Read the model definition and answer for the solid it produces. Units are mm, in the model's axes. A direction names the side the tool comes from. Give positions to 0.01 mm unless a question says otherwise; leave off trailing zeros. Order: outer loops, then holes, each group sorted by start corner. A loop starts at its lowest first (then second) coordinate and runs counter-clockwise, first axis right, second up. Notation, with made-up numbers: (-38.5, 2) -> (-1.5, 2) arc R24 ccw to (-1.5, 14) -> close; hole circle Ø6 at (-4, -15). An arc over 180 degrees is marked (long way). Answer as CSV lines item,"result". Start each with the question number.
1) Straight lines are drawn through the part: L1, parallel to X at y = 0, z = 48.5; L2, parallel to Y at x = 237.5, z = 21.5; L3, parallel to X at y = -32, z = 38. For each, find the intervals that lie inside material, in ascending order. Write a range as from..to.
2) Find section A-A (x = 0). Determine the outline of the cut face in (y, z), and give its area (3 significant figures).
3) The mould has two halves that part along Z. Classify faces 1 (the face through (278.814, 31.839, 41.915)), 2 (the face through (246, -25.4, 38)), 3 (the face through (284.86, -31.66, 20.34)): +Z half, -Z half, draft (parallel to the pull), parting line (faces both ways), or undercut.
4) Find section C-C (x = 228). Determine the outline of the cut face in (y, z), and give its area (3 significant figures).
5) Find section B-B (z = 6.5). Determine the outline of the cut face in (x, y).
6) For faces 4 (the face through (43.272, -16.365, 37.744)), 5 (the face through (237, 38.1, 38)), 6 (the face through (122, -23, 31.75)), 7 (the face through (215.9, 0, 38)), determine the directions among +Z, -Z, +X, -X, +Y, -Y from which every point of the face is accessible in a straight line to the end or side of a thin tool.
7) Find section D-D (y = -44.5). Determine the outline of the cut face in (x, z).
8) Flat-ended cylindrical pins translate along their axes: pin 1 Ø5 at (y, z) = (-10.5, 18.5) entering from -X; pin 2 Ø7.5 at (y, z) = (24.5, 28.5) entering from -X; pin 3 Ø15 at (y, z) = (3.5, 34.5) entering from +X. Find the tip coordinate at first contact, or state that the pin passes through.
```python
from build123d import *
from build123d import SkipClean  # not in build123d's __all__

# Parameters (mm, degrees)
F1_DEPTH    = 76.2
F3_DEPTH    = 12.7
F4_DEPTH    = 12.7
F5_T1_DEPTH = 50.8
F7_DEPTH    = 50.8
F8_R        = 25.39999
F9_R        = 12.7
F10_DEPTH   = 12.7
F13_DEPTH   = 38.1
F14_R       = 19.04999
F15_R       = 9.525
F16_DEPTH   = 12.7


# Not quite as in the source:
# - a fillet or chamfer that OpenCascade refuses, or shapes differently, is made with other operations: its cross-section is extruded or revolved along the edge and cut away or added
# - a fillet or chamfer is up to 0.001 mm smaller than in the source, because OpenCascade refuses the exact size


with BuildPart() as f1:
    # F0 (on Top) → F1 (new body)
    with BuildSketch(Plane.XY):
        with BuildLine():
            Line((-25.4, 0), (-38.1, 0))
            ThreePointArc((-38.1, 0), (-6.4427853895, -37.5513051228), (35.9210244843, -12.7))
            ThreePointArc((35.9210244843, -12.7), (37.5513051228, -6.4427853895), (38.1, 0))
            Line((38.1, 0), (25.4, 0))
            ThreePointArc((25.4, 0), (0, -25.4), (-25.4, 0))
        make_face()
        with BuildLine():
            ThreePointArc((38.1, 0), (37.5513051228, -6.4427853895), (35.9210244843, -12.7))
            Line((35.9210244843, -12.7), (203.2, -12.7))
            Line((203.2, -12.7), (203.2, 0))
            Line((203.2, 0), (38.1, 0))
        make_face()
    extrude(amount=F1_DEPTH)

    # F2 (on face) → F3 (cut)
    with BuildSketch(Plane.XY.offset(76.2)):
        with BuildLine():
            ThreePointArc((38.1, 0), (37.5513051228, -6.4427853895), (35.9210244843, -12.7))
            Line((35.9210244843, -12.7), (203.2, -12.7))
            Line((203.2, -12.7), (203.2, 0))
            Line((203.2, 0), (38.1, 0))
        make_face()
    extrude(amount=-F3_DEPTH, mode=Mode.SUBTRACT)

    # F0 (on Top) → F4 (cut)
    with BuildSketch(Plane.XY):
        with BuildLine():
            ThreePointArc((38.1, 0), (37.5513051228, -6.4427853895), (35.9210244843, -12.7))
            Line((35.9210244843, -12.7), (203.2, -12.7))
            Line((203.2, -12.7), (203.2, 0))
            Line((203.2, 0), (38.1, 0))
        make_face()
    extrude(amount=F4_DEPTH, mode=Mode.SUBTRACT)

    # F5: fillet of radius 50.8 on 1 edges, made by hand

    # F5_s2 → F5_t1 (join)
    with BuildSketch(Plane.XY.offset(12.7)):
        with BuildLine():
            ThreePointArc((62.2170394667, -12.7), (43.0164442378, -16.4683389316), (26.6644454857, -27.2142857143))
            ThreePointArc((26.6644454857, -27.2142857143), (32.1232219008, -20.4867912253), (35.9210244843, -12.7))
            Line((35.9210244843, -12.7), (62.2170394667, -12.7))
        make_face()
    extrude(amount=F5_T1_DEPTH)

    # F6 (on face) → F7 (join, through all)
    with BuildSketch(Plane.XY.offset(63.5)):
        Polygon((215.9, 0), (203.2, 0), (203.2, -12.7), (203.2, -38.1), (292.1, -38.1), (292.1, -25.4), (215.9, -25.4), align=None)
    extrude(amount=-F7_DEPTH)

    # F8 (radius 25.4 in the source; OpenCascade refuses exactly that, so slightly less here)
    f8_edges = [f1.edges().sort_by_distance(p)[0] for p in [
        (292.1, -31.75, 63.5),
        (292.1, -31.75, 12.7),
    ]]
    fillet(f8_edges, radius=F8_R)

    # F9 (on face) → F10 (cut, through all)
    with BuildSketch(Plane.XZ.offset(38.1)):
        with Locations((266.7, 38.1)):
            Circle(F9_R)
    extrude(amount=-F10_DEPTH, mode=Mode.SUBTRACT)

    # F11: F1 across plane


with BuildPart() as f1_1:
    add(f1.part, clean=False)
    with SkipClean():  # cleaning this boolean's faces spoils the solid; the shape is the same uncleaned
        add(f1.part.mirror(Plane.XZ), clean=False)

    # F12 (on face) → F13 (join)
    with BuildSketch(Plane.XZ.offset(12.7)):
        Polygon((146.05, 44.45), (127, 44.45), (107.95, 44.45), (107.95, 31.75), (127, 31.75), (146.05, 31.75), align=None)
    extrude(amount=F13_DEPTH)

    # F14 (radius 19.05 in the source; OpenCascade refuses exactly that, so slightly less here)
    f14_edges = [f1_1.edges().sort_by_distance(p)[0] for p in [
        (107.95, -50.8, 38.1),
        (146.05, -50.8, 38.1),
    ]]
    fillet(f14_edges, radius=F14_R)

    # F15 (on face) → F16 (cut, through all)
    with BuildSketch(Plane.XY.offset(44.45)):
        with Locations((127, -31.75)):
            Circle(F15_R)
    extrude(amount=-F16_DEPTH, mode=Mode.SUBTRACT)


solid = f1_1.part
```
Findings below:
1,L1,"-38.1..-25.4, 25.4..215.9"
1,L2,"-38.1..-25.4, 25.4..38.1"
1,L3,"-20.68..20.68, 107.95..117.48, 136.52..146.05, 203.2..254, 279.4..292.1"
2,outline,"(-38.1, 0) -> (-25.4, 0) -> (-25.4, 76.2) -> (-38.1, 76.2) -> close; (25.4, 0) -> (38.1, 0) -> (38.1, 76.2) -> (25.4, 76.2) -> close"
2,area,"1,940 mm²"
3,face 1,"undercut"
3,face 2,"draft"
3,face 3,"-Z half"
4,outline,"(-38.1, 12.7) -> (-25.4, 12.7) -> (-25.4, 63.5) -> (-38.1, 63.5) -> close; (25.4, 12.7) -> (38.1, 12.7) -> (38.1, 63.5) -> (25.4, 63.5) -> close"
4,area,"1,290 mm²"
5,outline,"circle Ø76.2 at (0, 0); hole circle Ø50.8 at (0, 0)"
6,face 4,"+Z, -Z, -Y"
6,face 5,"+Z, -Z, +X, -X, +Y"
6,face 6,"-Z, -Y"
6,face 7,"+Z, -Z, +X"
7,outline,"(112.85, 31.75) -> (141.15, 31.75) -> (141.15, 44.45) -> (112.85, 44.45) -> close"
8,pin 1,"x = -37.25"
8,pin 2,"x = -31.95"
8,pin 3,"x = 215.9"
